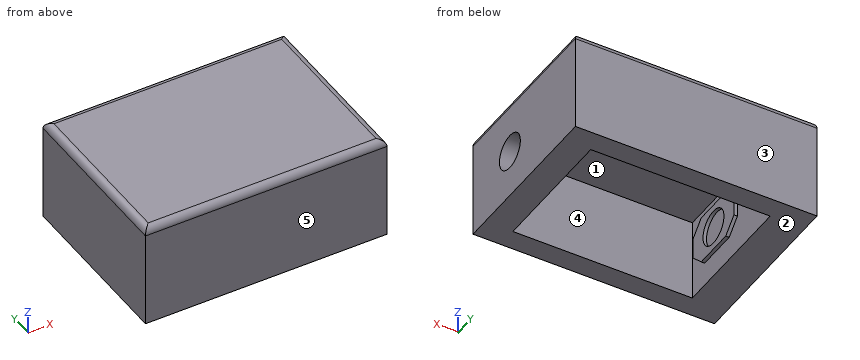
from build123d import *

# Parameters (mm, degrees)
F2_DEPTH = 150
F3_W     = 260
F3_H     = 190
F4_DEPTH = 120
F5_R     = 25.5
F6_DEPTH = 300
F7_R     = 10
F8_W     = 100
F8_H     = 70
F8_R     = 25.5
F9_DEPTH = 5
F10_SIZE = 20


with BuildPart() as f2:
    # F1 (on Top) → F2 (new body)
    with BuildSketch(Plane.XY):
        Polygon((173, -125), (175, -125), (175, 125), (-175, 125), (-175, -125), align=None)
    extrude(amount=-F2_DEPTH)

    # F3 (on face) → F4 (cut)
    with BuildSketch(Plane(origin=(0, 0, -150), x_dir=(1, 0, 0), z_dir=(0, 0, -1))):
        with Locations((5, 0)):
            Rectangle(F3_W, F3_H)
    extrude(amount=-F4_DEPTH, mode=Mode.SUBTRACT)

    # F5 (on face) → F6 (cut, through all)
    with BuildSketch(Plane.YZ.offset(175)):
        with Locations((-35, -80)):
            Circle(F5_R)
    extrude(amount=-F6_DEPTH, mode=Mode.SUBTRACT)

    # F7
    f7_edges = [f2.edges().sort_by_distance(p)[0] for p in [
        (0, -125, 0),
        (-175, 0, 0),
        (0, 125, 0),
        (175, 0, 0),
    ]]
    fillet(f7_edges, radius=F7_R)

    # F8 (on face) → F9 (join)
    with BuildSketch(Plane.YZ.offset(-125)):
        with Locations((-35, -80)):
            Rectangle(F8_W, F8_H)
        with Locations((-35, -80)):
            Circle(F8_R, mode=Mode.SUBTRACT)
    extrude(amount=F9_DEPTH)

    # F10
    f10_edges = [f2.edges().sort_by_distance(p)[0] for p in [
        (-122.5, -85, -115),
        (-122.5, -85, -45),
        (-122.5, 15, -115),
        (-122.5, 15, -45),
    ]]
    chamfer(f10_edges, length=F10_SIZE)


solid = f2.part
CAD build for the part. Positions are in the model's coordinates, mm. Face numbers are marked on the shaded views. A direction names the side the tool comes from. Coordinates: 2 decimals unless noted, no trailing zeros. Write each loop counter-clockwise with the first axis right and the second up, starting at its lowest first coordinate (ties: lowest second). Pieces come first, ordered by that corner, then holes. Notation, with made-up numbers: M -38.75,67.25 L -0.75,67.25 A30 ccw -0.75,89.25 Z; hole C -29.75,76.5 d8. An arc over 180 degrees is marked long. Answer as a JSON object with one key per item and string values. Group by question number.
1) Mould opens along Y. For the marked faces 1, 2 and 3 say: +Y half, -Y half, draft (parallel to the pull), parting line (faces both ways), or undercut.
2) Wall check: line 1 (Z direction, x = -122.95, y = -35); line 2 (Y direction, x = 36.5, z = -78); line 3 (X direction, y = 16, z = -78). Give the ranges that are in metal, low to high. Write a range as from..to.
3) Saw through at D-D (y = 35.5). Write the cut outline in (x, z), plus the area to 3 significant figures.
4) Tool access for the marked faces 4 and 5: list every direction of +Z, -Z, +X, -X, +Y, -Y with a clear straight run to the whole face (end or side of a thin tool).
5) Saw through at C-C (z = -80). Write the cut outline in (x, y), plus the area to 3 significant figures.
6) Saw through at B-B (x = 120). Write the cut outline in (y, z), plus the area to 3 significant figures.
7) Saw through at A-A (y = -35). Write the cut outline in (x, z).
8) Pin check, flat tips, straight feed: pin 1 Ø15.5 at (y, z) = (-36.5, -80.5) entering from +X; pin 2 Ø1 at (x, y) = (-62, -13.5) entering from -Z; pin 3 Ø1.5 at (x, y) = (-123, -29) entering from -Z. Stop position of each tip, or through.
Values follow:
{
 "1": {"face 1": "undercut", "face 2": "draft", "face 3": "+Y half"},
 "2": {"line 1": "z = -115..-105.5, -54.5..-45, -30..0", "line 2": "y = -125..-95, 95..125", "line 3": "x = -175..-125, 135..175"},
 "3": {"outline": "M -175,-150 L -125,-150 L -125,-30 L 135,-30 L 135,-150 L 175,-150 L 175,-10 A10 ccw 165,0 L -165,0 A10 ccw -175,-10 Z", "area": "21,300 mm2"},
 "4": {"face 4": "-Z", "face 5": "+Z, -Z, +X, -X, -Y"},
 "5": {"outline": "M -175,-125 L 175,-125 L 175,-60.5 L 135,-60.5 L 135,-95 L -125,-95 L -125,-85 L -120,-85 L -120,-60.5 L -125,-60.5 L -125,-9.5 L -120,-9.5 L -120,15 L -125,15 L -125,95 L 135,95 L 135,-9.5 L 175,-9.5 L 175,125 L -175,125 Z", "area": "36,300 mm2"},
 "6": {"outline": "M -125,-150 L -95,-150 L -95,-30 L 95,-30 L 95,-150 L 125,-150 L 125,-10 A10 ccw 115,0 L -115,0 A10 ccw -125,-10 Z", "area": "14,700 mm2"},
 "7": {"outline": "M -175,-150 L -125,-150 L -125,-115 L -120,-115 L -120,-105.5 L -125,-105.5 L -125,-54.5 L -120,-54.5 L -120,-45 L -125,-45 L -125,-30 L 135,-30 L 135,-54.5 L 175,-54.5 L 175,-10 A10 ccw 165,0 L -165,0 A10 ccw -175,-10 Z; M 135,-150 L 175,-150 L 175,-105.5 L 135,-105.5 Z"},
 "8": {"pin 1": "stops at x = -125", "pin 2": "stops at z = -30", "pin 3": "stops at z = -115"}
}
